from build123d import *

# Parameters (mm, degrees)
BARRA_START       = -44.75
SK_BARRA_W        = 13
SK_BARRA_H        = 74
BARRA_DEPTH       = 5
EXTREMOS_START    = -44.75
SK_EXTREMOS_R     = 6.5
EXTREMOS_DEPTH    = 8.65
PERNO_696_START   = -51.75
SK_PERNO_696_R    = 2.975
PERNO_696_DEPTH   = 7
PASANTES_M3_START = -44.75
SK_PASANTES_M3_R  = 1.7
PASANTES_M3_DEPTH = 8.65
CAJAS_M3_START    = -44.75
SK_CAJAS_M3_R     = 3
CAJAS_M3_DEPTH    = 6.85


with BuildPart() as part:
    # Sk_Barra → Barra (new body)
    with BuildSketch(Plane(origin=(0, 0, 0), x_dir=(1, 0, 0), z_dir=(0, 1, 0)).offset(BARRA_START)):
        with Locations((0, -170)):
            Rectangle(SK_BARRA_W, SK_BARRA_H)
    extrude(amount=BARRA_DEPTH)

    # Sk_Extremos → Extremos (add)
    with BuildSketch(Plane(origin=(0, 0, 0), x_dir=(1, 0, 0), z_dir=(0, 1, 0)).offset(EXTREMOS_START)):
        with Locations((0, -133)):
            Circle(SK_EXTREMOS_R)
        with Locations((0, -207)):
            Circle(SK_EXTREMOS_R)
    extrude(amount=EXTREMOS_DEPTH)

    # Sk_Perno_696 → Perno_696 (add)
    with BuildSketch(Plane(origin=(0, 0, 0), x_dir=(1, 0, 0), z_dir=(0, 1, 0)).offset(PERNO_696_START)):
        with Locations(Location((0, -170, 0), (0, 0, 270))):
            Circle(SK_PERNO_696_R)
    extrude(amount=PERNO_696_DEPTH)

    # Sk_Pasantes_M3 → Pasantes_M3 (cut)
    with BuildSketch(Plane(origin=(0, 0, 0), x_dir=(1, 0, 0), z_dir=(0, 1, 0)).offset(PASANTES_M3_START)):
        with Locations(Location((0, -133, 0), (0, 0, 270))):
            Circle(SK_PASANTES_M3_R)
        with Locations(Location((0, -207, 0), (0, 0, 270))):
            Circle(SK_PASANTES_M3_R)
    extrude(amount=PASANTES_M3_DEPTH, mode=Mode.SUBTRACT)

    # Sk_Cajas_M3 → Cajas_M3 (cut)
    with BuildSketch(Plane(origin=(0, 0, 0), x_dir=(1, 0, 0), z_dir=(0, 1, 0)).offset(CAJAS_M3_START)):
        with Locations(Location((0, -133, 0), (0, 0, 90))):
            Circle(SK_CAJAS_M3_R)
        with Locations(Location((0, -207, 0), (0, 0, 90))):
            Circle(SK_CAJAS_M3_R)
    extrude(amount=CAJAS_M3_DEPTH, mode=Mode.SUBTRACT)


solid = part.part
CAD build for the part. Positions are in the model's coordinates, mm. A direction names the side the tool comes from. Round coordinates to 2 decimals unless told otherwise and drop trailing zeros. Loops run counter-clockwise (first coordinate to the right, second up) from the corner with the lowest first, then second, coordinate; pieces in that order, holes last.
(1) Which spindle directions (+Z, -Z, +X, -X, +Y, -Y) get a long thin tool onto all of the face, cutting with end or side? Do faces 1 (the flat face through (6.5, -42, 171)), 2 (the cylindrical face through (-0.846, -39.524, 126.555)), 3 (the cylindrical face through (-1.14, -48.3, 172.75)). Say none if no direction does.
(2) Drop flat-ended pins along their axis: pin 1 (3 mm diameter, centred on x = -1, z = 208, fed in from -Y); pin 2 (1.5 mm diameter, centred on x = 1, z = 135.5, fed in from -Y); pin 3 (1 mm diameter, centred on x = -2.5, y = -41, fed in from +Z); pin 4 (3 mm diameter, centred on x = 1, y = -41, fed in from +Z). Give the stop position or say it passes through.
(3) Cut at C-C (z = 170). Give the cut face in (x, y) (3 decimals), plus the area to 3 significant figures.
(4) Cut at B-B (y = -43.5). Give the cut face in (x, z).
(5) Wall check: line 1 along Z through (x, y) = (0, -36.6); line 2 along X through (y, z) = (-39.5, 207); line 3 along X through (y, z) = (-37.45, 207). Give the ranges that are in metal, low to high.
(6) Cut at D-D (x = 4.75). Give the cut face in (y, z).
(7) Cut at A-A (x = 0). Give the cut face in (y, z) (3 decimals), plus the area to 3 significant figures.
(8) Two-plate mould, pull along X, no slides. Class faces 4 (the flat face through (1.4, -36.1, 208.4)), 5 (the cylindrical face through (2.999, -39.524, 212.767)), 6 (the flat face through (2, -37.9, 133)): +X half, -X half, draft (parallel to the pull), parting line (faces both ways), or undercut.
Findings below:
1. face 1: +Z, -Z, +X, +Y, -Y
1. face 2: +Y
1. face 3: -Y
2. pin 1: stops at y = -37.9
2. pin 2: stops at y = -44.75
2. pin 3: stops at z = 213.18
2. pin 4: stops at z = 213.5
3. outline: (-6.5, -44.75) - (-2.975, -44.75) - (-2.975, -51.75) - (2.975, -51.75) - (2.975, -44.75) - (6.5, -44.75) - (6.5, -39.75) - (-6.5, -39.75) - close
3. area: 107 mm2
4. outline: (-6.5, 133) arc R6.5 ccw to (6.5, 133) - (6.5, 207) arc R6.5 ccw to (-6.5, 207) - close; hole circle Ø6 at (0, 133); hole circle Ø6 at (0, 207)
5. line 1: z = 126.5 to 131.3, 134.7 to 139.5, 200.5 to 205.3, 208.7 to 213.5
5. line 2: x = -6.5 to -3, 3 to 6.5
5. line 3: x = -6.5 to -1.7, 1.7 to 6.5
6. outline: (-44.75, 128.56) - (-36.1, 128.56) - (-36.1, 137.44) - (-39.75, 137.44) - (-39.75, 202.56) - (-36.1, 202.56) - (-36.1, 211.44) - (-44.75, 211.44) - close
7. outline: (-51.75, 167.025) - (-44.75, 167.025) - (-44.75, 136) - (-37.9, 136) - (-37.9, 134.7) - (-36.1, 134.7) - (-36.1, 139.5) - (-39.75, 139.5) - (-39.75, 200.5) - (-36.1, 200.5) - (-36.1, 205.3) - (-37.9, 205.3) - (-37.9, 204) - (-44.75, 204) - (-44.75, 172.975) - (-51.75, 172.975) - close; (-44.75, 126.5) - (-36.1, 126.5) - (-36.1, 131.3) - (-37.9, 131.3) - (-37.9, 130) - (-44.75, 130) - close; (-44.75, 210) - (-37.9, 210) - (-37.9, 208.7) - (-36.1, 208.7) - (-36.1, 213.5) - (-44.75, 213.5) - close
7. area: 477 mm2
8. face 4: draft
8. face 5: parting line
8. face 6: undercut
